Source: CAD feature listing. Evaluate the final solid. Frame: model axes, mm. A direction names the side the tool comes from. Round coordinates to 2 decimals unless told otherwise and drop trailing zeros. Write each loop counter-clockwise with the first axis right and the second up, starting at its lowest first coordinate (ties: lowest second). Pieces come first, ordered by that corner, then holes.
from build123d import *

# Parameters (mm, degrees)
SKETCH1_W            = 58
SKETCH1_H            = 40
BOSS_EXTRUDE1_DEPTH  = 1
SKETCH2_W            = 14
SKETCH2_H            = 13
BOSS_EXTRUDE2_DEPTH  = 1
SKETCH3_W            = 3
SKETCH3_H            = 10
CUT_EXTRUDE1_DEPTH   = 1
SKETCH4_W            = 12.5
SKETCH4_H            = 11.5
SKETCH4_W_2          = 15
SKETCH4_H_2          = 15
BOSS_EXTRUDE3_DEPTH  = 1
SKETCH5_W            = 13
SKETCH5_H            = 6
BOSS_EXTRUDE4_DEPTH  = 2.6
CUT_EXTRUDE2_DEPTH   = 5
SKETCH7_W            = 21.3
SKETCH7_H            = 7.2
BOSS_EXTRUDE5_DEPTH  = 2.5
SKETCH8_W            = 17.3
SKETCH8_H            = 3.2
CUT_EXTRUDE3_DEPTH   = 1
SKETCH9_R            = 1.6
CUT_EXTRUDE4_DEPTH   = 2
SKETCH10_W           = 9
SKETCH10_H           = 5
BOSS_EXTRUDE6_DEPTH  = 3.6
SKETCH11_W           = 12.5
SKETCH11_H           = 6.25
BOSS_EXTRUDE7_DEPTH  = 5
SKETCH12_W           = 10
SKETCH12_H           = 10
BOSS_EXTRUDE8_DEPTH  = 2.5
SKETCH13_R           = 1
SKETCH13_R_2         = 0.8
BOSS_EXTRUDE9_DEPTH  = 1
SKETCH14_R           = 0.15
BOSS_EXTRUDE10_DEPTH = 1


with BuildPart() as part:
    # Sketch1 → Boss-Extrude1 (new body)
    with BuildSketch(Plane(origin=(0, 0, 0), x_dir=(1, 0, 0), z_dir=(0, 1, 0))):
        Rectangle(SKETCH1_W, SKETCH1_H)
    extrude(amount=BOSS_EXTRUDE1_DEPTH)

    # Sketch2 → Boss-Extrude2 (add)
    with BuildSketch(Plane(origin=(0, 1, 0), x_dir=(1, 0, 0), z_dir=(0, 1, 0))):
        with Locations((-21, -3.5)):
            Rectangle(SKETCH2_W, SKETCH2_H)
    extrude(amount=BOSS_EXTRUDE2_DEPTH)

    # Sketch3 → Cut-Extrude1 (cut)
    with BuildSketch(Plane(origin=(0, 2, 0), x_dir=(1, 0, 0), z_dir=(0, 1, 0))):
        with Locations((-26.5, -3)):
            Rectangle(SKETCH3_W, SKETCH3_H)
    extrude(amount=-CUT_EXTRUDE1_DEPTH, mode=Mode.SUBTRACT)

    # Sketch4 → Boss-Extrude3 (add)
    with BuildSketch(Plane(origin=(0, 1, 0), x_dir=(1, 0, 0), z_dir=(0, 1, 0))):
        with Locations((-5.25, -4.95)):
            Rectangle(SKETCH4_W, SKETCH4_H)
        with Locations((12.5, -6)):
            Rectangle(SKETCH4_W_2, SKETCH4_H_2)
    extrude(amount=BOSS_EXTRUDE3_DEPTH)

    # Sketch5 → Boss-Extrude4 (add)
    with BuildSketch(Plane(origin=(0, 1, 0), x_dir=(1, 0, 0), z_dir=(0, 1, 0))):
        with Locations((8.5, -18.3)):
            Rectangle(SKETCH5_W, SKETCH5_H)
    extrude(amount=BOSS_EXTRUDE4_DEPTH)

    # Sketch6 → Cut-Extrude2 (cut)
    with BuildSketch(Plane.XY.offset(21.3)):
        Polygon((2.25, 3.35), (14.75, 3.35), (14.75, 1.25), (9.95, 1.25), (9.25, 1.95), (8.55, 1.25), (2.25, 1.25), align=None)
    extrude(amount=-CUT_EXTRUDE2_DEPTH, mode=Mode.SUBTRACT)

    # Sketch7 → Boss-Extrude5 (add)
    with BuildSketch(Plane(origin=(0, 1, 0), x_dir=(1, 0, 0), z_dir=(0, 1, 0))):
        with Locations((-11.6, -15.4)):
            Rectangle(SKETCH7_W, SKETCH7_H)
    extrude(amount=BOSS_EXTRUDE5_DEPTH)

    # Sketch8 → Cut-Extrude3 (cut)
    with BuildSketch(Plane(origin=(0, 3.5, 0), x_dir=(1, 0, 0), z_dir=(0, 1, 0))):
        Polygon((-21.75, -12.3), (-21.75, -16.586355197), (-19.749371343, -18.5), (-1.45, -18.5), (-1.45, -12.3), align=None)
        with Locations((-11.6, -15.4)):
            Rectangle(SKETCH8_W, SKETCH8_H, mode=Mode.SUBTRACT)
    extrude(amount=-CUT_EXTRUDE3_DEPTH, mode=Mode.SUBTRACT)

    # Sketch9 → Cut-Extrude4 (cut, through all)
    with BuildSketch(Plane(origin=(0, 1, 0), x_dir=(1, 0, 0), z_dir=(0, 1, 0))):
        with Locations((-26.5, 17.5)):
            Circle(SKETCH9_R)
        with Locations((20, 17.5)):
            Circle(SKETCH9_R)
        with Locations((20, -17.5)):
            Circle(SKETCH9_R)
        with Locations((-26.5, -17.5)):
            Circle(SKETCH9_R)
    extrude(amount=-CUT_EXTRUDE4_DEPTH, mode=Mode.SUBTRACT)

    # Sketch10 → Boss-Extrude6 (add)
    with BuildSketch(Plane.XZ):
        with Locations((-18.5, 18.5)):
            Rectangle(SKETCH10_W, SKETCH10_H)
        with Locations((-5.5, 18.5)):
            Rectangle(SKETCH10_W, SKETCH10_H)
        with Locations((-17.8, -18.5)):
            Rectangle(SKETCH10_W, SKETCH10_H)
        with Locations((-4.8, -18.5)):
            Rectangle(SKETCH10_W, SKETCH10_H)
    extrude(amount=BOSS_EXTRUDE6_DEPTH)

    # Sketch11 → Boss-Extrude7 (add)
    with BuildSketch(Plane.XZ):
        with Locations((10.25, -20.475)):
            Rectangle(SKETCH11_W, SKETCH11_H)
    extrude(amount=BOSS_EXTRUDE7_DEPTH)

    # Sketch12 → Boss-Extrude8 (add)
    with BuildSketch(Plane.XZ):
        with Locations((-18, 6.5)):
            Rectangle(SKETCH12_W, SKETCH12_H)
    extrude(amount=BOSS_EXTRUDE8_DEPTH)

    # Sketch13 → Boss-Extrude9 (add)
    with BuildSketch(Plane.XZ):
        with Locations((-26.5, 12.5)):
            Circle(SKETCH13_R)
        with Locations((-26.5, 12.5)):
            Circle(SKETCH13_R_2, mode=Mode.SUBTRACT)
        with Locations((-26.5, 4)):
            Circle(SKETCH13_R)
        with Locations((-26.5, 4)):
            Circle(SKETCH13_R_2, mode=Mode.SUBTRACT)
        with Locations((-26.5, -3.5)):
            Circle(SKETCH13_R)
        with Locations((-26.5, -3.5)):
            Circle(SKETCH13_R_2, mode=Mode.SUBTRACT)
    extrude(amount=BOSS_EXTRUDE9_DEPTH)

    # Sketch14 → Boss-Extrude10 (add)
    with BuildSketch(Plane.XZ):
        with Locations((-26.5, 12.5)):
            Circle(SKETCH14_R)
        with Locations((-26.5, 4)):
            Circle(SKETCH14_R)
        with Locations((-26.5, -3.5)):
            Circle(SKETCH14_R)
    extrude(amount=BOSS_EXTRUDE10_DEPTH)


solid = part.part
1) Pull-direction query (Y, two-part tool) for faces 6 (the face through (-27.237, -0.493, 4.676)), 7 (the face through (12, 1.25, 19)), 8 (the face through (8, 3.6, 18)); classes: released by +Y, released by -Y, zero draft, split by the parting line, or undercut.
Taken from the geometry:
face 6: zero draft
face 7: undercut
face 8: released by +Y
2) Section query A-A on x = -4.5. Return the cut outline in (y, z).
Taken from the geometry:
outline: (-3.6, -21) - (0, -21) - (0, -20) - (1, -20) - (1, -0.8) - (2, -0.8) - (2, 10.7) - (1, 10.7) - (1, 11.8) - (3.5, 11.8) - (3.5, 12.3) - (2.5, 12.3) - (2.5, 13.8) - (3.5, 13.8) - (3.5, 17) - (2.5, 17) - (2.5, 18.5) - (3.5, 18.5) - (3.5, 19) - (1, 19) - (1, 20) - (0, 20) - (0, 21) - (-3.6, 21) - (-3.6, 16) - (0, 16) - (0, -16) - (-3.6, -16) - close
3) Section query C-C on z = 0. Return the cut outline in (x, y), then the cut area to 3 significant figures.
Taken from the geometry:
outline: (-29, 0) - (29, 0) - (29, 1) - (20, 1) - (20, 2) - (5, 2) - (5, 1) - (1, 1) - (1, 2) - (-11.5, 2) - (-11.5, 1) - (-14, 1) - (-14, 2) - (-25, 2) - (-25, 1) - (-29, 1) - close
area: 96.5 mm2
4) Section query B-B on z = 14.5. Return the cut outline in (x, y).
Taken from the geometry:
outline: (-29, 0) - (29, 0) - (29, 1) - (-0.95, 1) - (-0.95, 3.5) - (-1.45, 3.5) - (-1.45, 2.5) - (-2.95, 2.5) - (-2.95, 3.5) - (-20.25, 3.5) - (-20.25, 2.5) - (-21.75, 2.5) - (-21.75, 3.5) - (-22.25, 3.5) - (-22.25, 1) - (-29, 1) - close
5) Section query D-D on x = 24. Return the cut outline in (y, z), then the cut area to 3 significant figures.
Taken from the geometry:
outline: (0, -20) - (1, -20) - (1, 20) - (0, 20) - close
area: 40.0 mm2
6) Contact query for flat-ended pins moving along their axis: P1, Ø1.5, axis at y = -3, z = -22, coming from the +X side; P2, Ø3, axis at x = 18.5, z = -7, coming from the -Y side; P3, Ø8, axis at x = -20, z = -18.5, coming from the -Y side. Output: stop coordinate, or through.
Taken from the geometry:
P1: stops at x = 16.5
P2: stops at y = 0
P3: stops at y = -3.6
7) Material intervals for line 1 (X direction, y = 0.4, z = -17.5); line 2 (Z direction, x = -26.5, y = 0.75); line 3 (X direction, y = 3.25, z = 15), sorted ascending.
Taken from the geometry:
line 1: x = -29 to -28.1, -24.9 to 18.4, 21.6 to 29
line 2: z = -20 to -19.1, -15.9 to 15.9, 19.1 to 20
line 3: x = -22.25 to -21.75, -20.25 to -2.95, -1.45 to -0.95
8) Reachability of faces 1 (the face through (-18, -1, 11.5)), 2 (the face through (-20, 2, 3)), 3 (the face through (-27, 0, 4)), 4 (the face through (-9.3, -2, -19)), 5 (the face through (-19, -2, 16)) from +Z, -Z, +X, -X, +Y, -Y: full face, straight path, thin tool, end or side. Return the list, or none.
Taken from the geometry:
face 1: +X, -Y
face 2: -Z, +X, -X, +Y
face 3: -Y
face 4: -Z, -Y
face 5: +X, -X, -Y
